Verification items for the finished model (mm, model axes). Face numbers are marked on the shaded views. A direction names the side the tool comes from. Coordinates: 2 decimals unless noted, no trailing zeros. Loops run counter-clockwise (first coordinate to the right, second up) from the corner with the lowest first, then second, coordinate; pieces in that order, holes last.
Q1. Mould release check, pull along Y, two halves, no side actions. Record for the marked faces 6, 7 and 8: +Y half, -Y half, draft (parallel to the pull), parting line (faces both ways), or undercut.
Q2. Sectioned sample at D-D (z = 2.5). Enter the section's corners in (x, y).
Q3. Sectioned sample at B-B (y = 3.25). Enter the section's corners in (x, z).
Q4. Go/stop test with flat-tipped pins: P1, Ø5, axis at y = -7.5, z = -3, coming from the -X side; P2, Ø4, axis at x = 1.5, y = -6, coming from the +Z side; P3, Ø1.6, axis at x = 5, z = -7, coming from the -Y side. Record where each tip stops, or that it passes through.
Q5. Sectioned sample at C-C (x = 5.5). Enter the section's corners in (y, z), then the cut area to 3 significant figures.
Q6. Sectioned sample at A-A (z = -7). Enter the section's corners in (x, y).
Q7. Material ranges on probe 1 along X at (y, z) = (5, 4.5); probe 2 along Z at (x, y) = (0.75, -7.25); probe 3 along Y at (x, z) = (2, 1), recorded low to high.
Q8. Access from +Z, -Z, +X, -X, +Y, -Y to the whole of each face (thin tool, end or side, straight path). Record for the marked faces 1, 2, 3, 4 and 5.
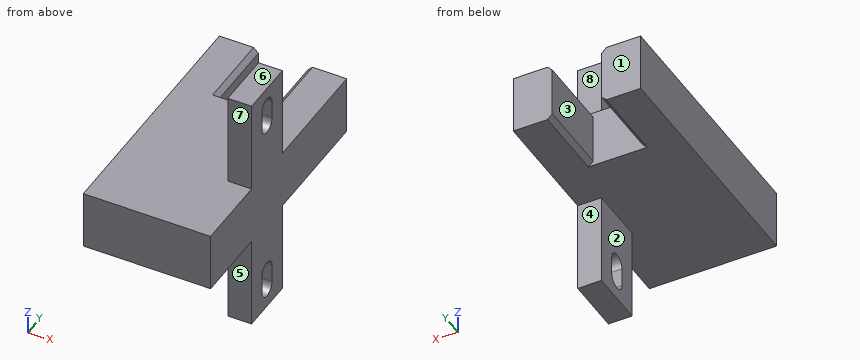
```python
from build123d import *

# Parameters (mm, degrees)
EXTRUDE_1_DEPTH     = 6.2
SKETCH_2_W          = 2.5
SKETCH_2_H          = 6
EXTRUDE_2_DEPTH     = 9.8
SKETCH_3_W          = 2.5
SKETCH_3_H          = 6
EXTRUDE_3_DEPTH     = 9.8
CUT_EXTRUDE_1_DEPTH = 28.432848917
CHAMFER_1_SIZE      = 0.5


with BuildPart() as part:
    # 草图1 → 凸台-拉伸1 (new body)
    with BuildSketch(Plane.XY):
        Polygon((2.6, 0.795472494), (-2.6, 0.795472494), (-2.6, 8.795472494), (-6.7, 8.795472494), (-6.7, -17.804527506), (6.7, -17.804527506), (6.7, 8.795472494), (2.6, 8.795472494), align=None)
    extrude(amount=EXTRUDE_1_DEPTH)

    # 草图2 → 凸台-拉伸2 (add)
    with BuildSketch(Plane.XY.offset(6.2)):
        with Locations((5.45, -6.804527506)):
            Rectangle(SKETCH_2_W, SKETCH_2_H)
    extrude(amount=EXTRUDE_2_DEPTH)

    # 草图3 → 凸台-拉伸3 (add)
    with BuildSketch(Plane(origin=(0, 0, 0), x_dir=(-1, 0, 0), z_dir=(0, 0, -1))):
        with Locations((-5.45, -6.804527506)):
            Rectangle(SKETCH_3_W, SKETCH_3_H)
    extrude(amount=EXTRUDE_3_DEPTH)

    # 草图5 → 切除-拉伸1 (cut, through all)
    with BuildSketch(Plane(origin=(6.7, 0, 0), x_dir=(0, 0, -1), z_dir=(1, 0, 0))):
        with BuildLine():
            Line((-13.775713177, -5.804527506), (-11.824286823, -5.804527506))
            ThreePointArc((-11.824286823, -5.804527506), (-10.824286823, -6.804527506), (-11.824286823, -7.804527506))
            Line((-11.824286823, -7.804527506), (-13.775713177, -7.804527506))
            ThreePointArc((-13.775713177, -7.804527506), (-14.775713177, -6.804527506), (-13.775713177, -5.804527506))
        make_face()
        with BuildLine():
            Line((7.575713177, -5.804527506), (5.624286823, -5.804527506))
            ThreePointArc((5.624286823, -5.804527506), (4.624286823, -6.804527506), (5.624286823, -7.804527506))
            Line((5.624286823, -7.804527506), (7.575713177, -7.804527506))
            ThreePointArc((7.575713177, -7.804527506), (8.575713177, -6.804527506), (7.575713177, -5.804527506))
        make_face()
    extrude(amount=-CUT_EXTRUDE_1_DEPTH, mode=Mode.SUBTRACT)

    # 倒角1
    chamfer_1_edges = [part.edges().sort_by_distance(p)[0] for p in [
        (-2.6, 4.795472494, 0),
        (2.6, 4.795472494, 0),
        (-2.6, 4.795472494, 6.2),
        (2.6, 4.795472494, 6.2),
    ]]
    chamfer(chamfer_1_edges, length=CHAMFER_1_SIZE)


solid = part.part
```
Geometry check:
1. face 6: draft
1. face 7: -Y half
1. face 8: +Y half
2. outline: (-6.7, -17.8) - (6.7, -17.8) - (6.7, 8.8) - (2.6, 8.8) - (2.6, 0.8) - (-2.6, 0.8) - (-2.6, 8.8) - (-6.7, 8.8) - close
3. outline: (-6.7, 0) - (-3.1, 0) - (-2.6, 0.5) - (-2.6, 5.7) - (-3.1, 6.2) - (-6.7, 6.2) - close; (2.6, 0.5) - (3.1, 0) - (6.7, 0) - (6.7, 6.2) - (3.1, 6.2) - (2.6, 5.7) - close
4. P1: stops at x = 4.2
4. P2: stops at z = 6.2
4. P3: stops at y = -9.8
5. outline: (-17.8, 0) - (-9.8, 0) - (-9.8, -9.8) - (-3.8, -9.8) - (-3.8, 0) - (8.8, 0) - (8.8, 6.2) - (-3.8, 6.2) - (-3.8, 16) - (-9.8, 16) - (-9.8, 6.2) - (-17.8, 6.2) - close; hole (-7.8, -7.58) arc R1 ccw to (-5.8, -7.58) - (-5.8, -5.62) arc R1 ccw to (-7.8, -5.62) - close; hole (-7.8, 11.82) arc R1 ccw to (-5.8, 11.82) - (-5.8, 13.78) arc R1 ccw to (-7.8, 13.78) - close
5. area: 268 mm2
6. outline: (4.2, -9.8) - (6.7, -9.8) - (6.7, -7.8) - (4.2, -7.8) - close; (4.2, -5.8) - (6.7, -5.8) - (6.7, -3.8) - (4.2, -3.8) - close
7. probe 1: x = -6.7 to -2.6, 2.6 to 6.7
7. probe 2: z = 0 to 6.2
7. probe 3: y = -17.8 to 0.8
8. face 1: +Z, -Z, +X, -X, +Y
8. face 2: -Z, -X, +Y, -Y
8. face 3: +Z, -Z, +Y
8. face 4: -Z, +X, -X, +Y
8. face 5: -Z, +X, -X, -Y
